Work out the finished part from the listing and answer in its coordinate system (mm). A direction names the side the tool comes from. Give positions to 0.01 mm unless a question says otherwise; leave off trailing zeros. Loops run counter-clockwise (first coordinate to the right, second up) from the corner with the lowest first, then second, coordinate; pieces in that order, holes last. Notation, with made-up numbers: (30, 35.5) - (36, 35.5) arc R29 cw to (36, 62.5) - close; hole circle Ø1 at (50, 11.25). An arc over 180 degrees is marked (long way). One line per question, with ' | ' between items. Start each with the question number.
1. For a pull along Y with two mould halves and no side action, classify faces 4 (the face through (1.086, -13.299, -0.056)), 5 (the face through (-1.084, -32.181, 0.413)), 6 (the face through (2, -18, 7)) as released by +Y, released by -Y, zero draft, split by the parting line, or undercut.
2. Each of these flat-tipped pins is pushed along its axis until it touches: pin 1 (2 mm diameter, centred on x = -1, y = -4, fed in from +Z); pin 2 (2 mm diameter, centred on x = -0.5, y = -14.5, fed in from -Z). Where does it stop, or does it pass through?
3. Section B-B (z = -18) is taken. Determine the outline of the cut face in (x, y).
4. Section D-D (y = -22) is taken. Determine the outline of the cut face in (x, z), plus the area to 3 significant figures.
5. Section A-A (z = -2) is taken. Determine the outline of the cut face in (x, y) (3 decimals).
6. Find the intervals of material crossed by line 1 (Z direction, x = 1.4, y = -15); line 2 (Z direction, x = 0.3, y = -6); line 3 (Z direction, x = -0.35, y = -1), in increasing order.
7. Section C-C (y = -8.5) is taken. Determine the outline of the cut face in (x, z), plus the area to 3 significant figures.
8. Which of the six approach directions +Z, -Z, +X, -X, +Y, -Y give full straight-line access (tool end or side, diameter ignored) to faces 1 (the face through (-0.417, -17.052, 0.056)), 2 (the face through (-1.044, -21.727, 0.056)), 3 (the face through (-2, -14, 0))?
from build123d import *

# Parameters (mm, degrees)
BOSS_EXTRUDE1_DEPTH = 29.5
SKETCH3_4_R         = 2
BOSS_EXTRUDE2_DEPTH = 35
FILLET1_R           = 1
FILLET2_R           = 0.25
SKETCH4_R           = 3.5
CUT_EXTRUDE1_DEPTH  = 4
SKETCH5_R           = 0.75
BOSS_EXTRUDE3_DEPTH = 5
FILLET3_R           = 20


with BuildPart() as part:
    # Sketch3 → Boss-Extrude1 (new, symmetric)
    with BuildSketch(Plane.XY):
        with BuildLine():
            Line((2, -36), (2, 0))
            ThreePointArc((2, 0), (0, -2), (-2, 0))
            Line((-2, 0), (-2, -28))
            ThreePointArc((-2, -28), (-0.94427191, -32.472135955), (2, -36))
        make_face()
    extrude(amount=BOSS_EXTRUDE1_DEPTH, both=True)

    # Sketch3<4> → Boss-Extrude2 (add, symmetric)
    with BuildSketch(Plane.XY):
        Circle(SKETCH3_4_R)
    extrude(amount=BOSS_EXTRUDE2_DEPTH, both=True)

    # Fillet1
    fillet1_edges = [part.edges().sort_by_distance(p)[0] for p in [
        (-2, 0, -35),
        (-2, 0, 35),
    ]]
    fillet(fillet1_edges, radius=FILLET1_R)

    # Fillet2
    fillet2_edges = [part.edges().sort_by_distance(p)[0] for p in [
        (2, -36, 0),
    ]]
    fillet(fillet2_edges, radius=FILLET2_R)

    # Sketch4 → Cut-Extrude1 (cut, symmetric)
    with BuildSketch(Plane.XY):
        with Locations((2, -20)):
            Circle(SKETCH4_R)
    extrude(amount=CUT_EXTRUDE1_DEPTH, both=True, mode=Mode.SUBTRACT)

    # Sketch5 → Boss-Extrude3 (add, symmetric)
    with BuildSketch(Plane.XY):
        with Locations((1.25, -20)):
            Circle(SKETCH5_R)
    extrude(amount=BOSS_EXTRUDE3_DEPTH, both=True)

    # Chamfer1
    # the kernel refuses this chamfer: 10 mm, written as the material it takes off along each edge
    with BuildSketch(Plane(origin=(2, -16.5, -4), x_dir=(0.024228479876225433, 0.9997064472948483, 0), z_dir=(0, 0, 1))) as chamfer1_piece_1:
        with BuildLine():
            Line((5.944098049, 0), (-1.587763168, 2.698932243))
            Line((-1.587763168, 2.698932243), (-1.718492524, 2.54757229))
            ThreePointArc((-1.718492524, 2.54757229), (-0.583435154, 1.461046885), (-0.199941289, -0.004845696))
            Line((-0.199941289, -0.004845696), (0.004845696, -0.199941289))
            ThreePointArc((0.004845696, -0.199941289), (2.975150071, -0.127954198), (5.948943745, -0.199941289))
            Line((5.948943745, -0.199941289), (5.944098049, 0))
        make_face()
    extrude(amount=8, mode=Mode.SUBTRACT)

    # Fillet3
    fillet3_edges = [part.edges().sort_by_distance(p)[0] for p in [
        (-0.592592593, -17.648731481, 0),
    ]]
    fillet(fillet3_edges, radius=FILLET3_R)


solid = part.part
Conclusion:
1) face 4: undercut | face 5: released by -Y | face 6: zero draft
2) pin 1: z = 29.5 | pin 2: z = -29.5
3) outline: (-2, -28) arc R10 ccw to (1.59, -35.68) arc R0.25 ccw to (2, -35.48) - (2, 0) arc R2 ccw to (-2, 0) - close
4) outline: (-2, -29.5) - (2, -29.5) - (2, -4) - (-0.87, -4) - (-0.87, 4) - (2, 4) - (2, 29.5) - (-2, 29.5) - close | area: 213 mm²
5) outline: (-2, -28) arc R10 ccw to (1.59, -35.675) arc R0.25 ccw to (2, -35.483) - (2, -23.5) arc R3.5 cw to (-1.055, -18.292) arc R20 ccw to (0.147, -15.733) - (2, -10.931) - (2, 0) arc R2 ccw to (-2, 0) - close; circle Ø1.5 at (1.25, -20)
6) line 1: -29.5 to -4, 4 to 29.5 | line 2: -29.5 to 29.5 | line 3: -35 to 35
7) outline: (-2, -29.5) - (2, -29.5) - (2, 29.5) - (-2, 29.5) - close | area: 236 mm²
8) face 1: +X | face 2: none | face 3: +Z, -Z, -X, +Y, -Y
